Print and shaded views of the part. All mm, measured from the part's lowest x, y and z. A direction names the side the tool comes from. Round coordinates to 2 decimals unless told otherwise and drop trailing zeros. Loops run counter-clockwise (first coordinate to the right, second up) from the corner with the lowest first, then second, coordinate; pieces in that order, holes last. Notation, with made-up numbers: (-7.5, 77.25) -> (33.5, 77.25) arc R8 cw to (33.5, 82.25) -> close; hole circle Ø2 at (-39.75, 26). An arc over 180 degrees is marked (long way). Answer as CSV lines item,"result".
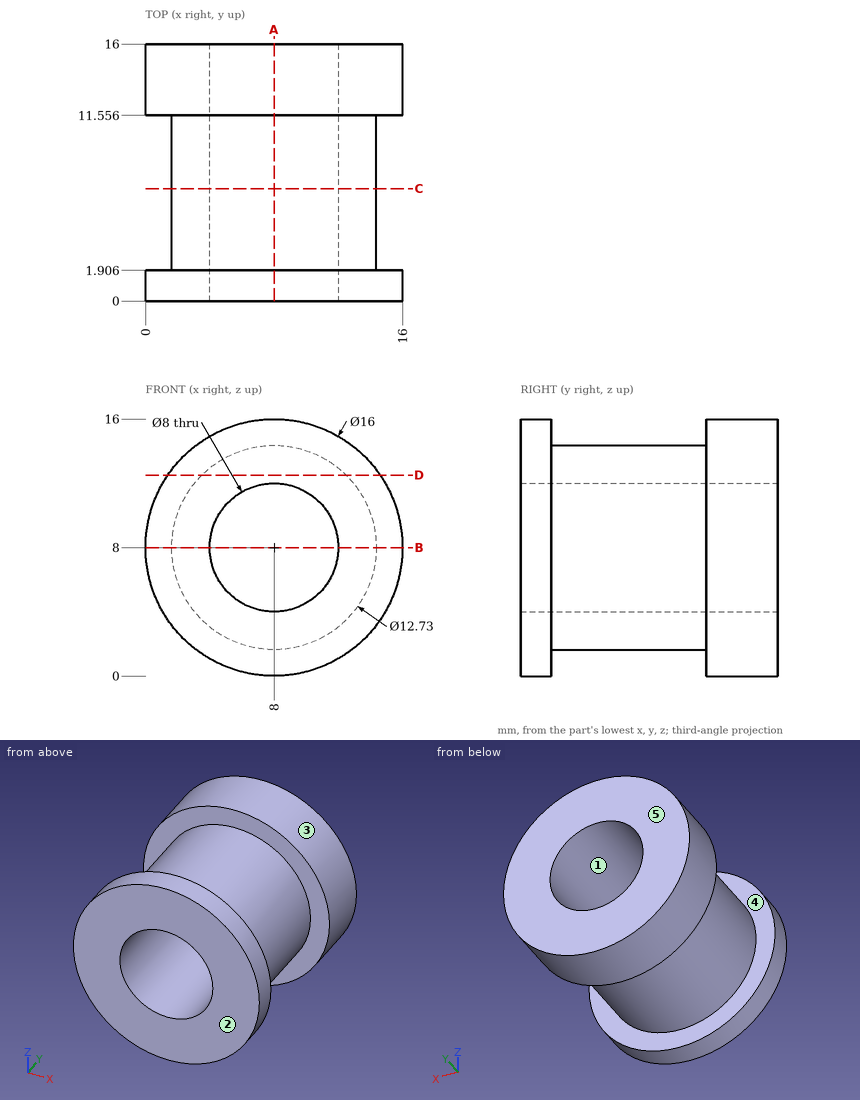
Q1. Drill centre lines: line 1 along X through (y, z) = (4.5, 8) (3 decimals); line 2 along Z through (x, y) = (8, 12). Where is each one in solid material? Low to high.
Geometry results:
line 1,"1.635 to 4, 12 to 14.365"
line 2,"0 to 4, 12 to 16"
Q2. Two-plate mould, pull along Z, no slides. Class the marked faces 1, 2 and 3: pulls with the +Z half, pulls with the -Z half, needs draft (parallel to the pull), parting line crosses it, or undercut.
Geometry results:
face 1,"undercut"
face 2,"needs draft"
face 3,"parting line crosses it"
Q3. Saw through at D-D, the plane z = 12.5. Write the cut outline in (x, y), then the cut area to 3 significant figures.
Geometry results:
outline,"(1.39, 0) -> (14.61, 0) -> (14.61, 1.91) -> (12.5, 1.91) -> (12.5, 11.56) -> (14.61, 11.56) -> (14.61, 16) -> (1.39, 16) -> (1.39, 11.56) -> (3.5, 11.56) -> (3.5, 1.91) -> (1.39, 1.91) -> close"
area,"171 mm2"
Q4. Saw through at C-C, the plane y = 7. Write the cut outline in (x, z) (3 decimals), then the cut area to 3 significant figures.
Geometry results:
outline,"circle Ø12.73 at (8, 8); hole circle Ø8 at (8, 8)"
area,"77.0 mm2"
Q5. Drop flat-ended pins along their axis: P1, Ø3, axis at y = 7, z = 9.5, coming from the +X side (3 decimals); P2, Ø1, axis at y = 11, z = 5, coming from the -X side; P3, Ø6, axis at y = 6.5, z = 7, coming from the -X side (3 decimals); P4, Ø4, axis at x = 8, z = 9, coming from the -Y side. Give the stop position or say it passes through.
Geometry results:
P1,"x = 14.365"
P2,"x = 2.15"
P3,"x = 1.635"
P4,"through"
Q6. Saw through at B-B, the plane z = 8. Write the cut outline in (x, y) (3 decimals).
Geometry results:
outline,"(0, 0) -> (4, 0) -> (4, 16) -> (0, 16) -> (0, 11.556) -> (1.635, 11.556) -> (1.635, 1.906) -> (0, 1.906) -> close; (12, 0) -> (16, 0) -> (16, 1.906) -> (14.365, 1.906) -> (14.365, 11.556) -> (16, 11.556) -> (16, 16) -> (12, 16) -> close"
Q7. Which spindle directions (+Z, -Z, +X, -X, +Y, -Y) get a long thin tool onto all of the face, cutting with end or side? Do the marked faces 4 and 5. Say none if no direction does.
Geometry results:
face 4,"none"
face 5,"+Z, -Z, +X, -X, +Y"
Q8. Saw through at A-A, the plane x = 8. Write the cut outline in (y, z) (3 decimals).
Geometry results:
outline,"(0, 0) -> (1.906, 0) -> (1.906, 1.635) -> (11.556, 1.635) -> (11.556, 0) -> (16, 0) -> (16, 4) -> (0, 4) -> close; (0, 12) -> (16, 12) -> (16, 16) -> (11.556, 16) -> (11.556, 14.365) -> (1.906, 14.365) -> (1.906, 16) -> (0, 16) -> close"
